Autodesk Inventor part; units mm, degrees
ref_plane "Work Plane1" through (30, 0, 0) normal (0, -0.5, 0.866) x (1, 0, 0)
ref_plane "YZ Plane" through (0, 0, 0) normal (1, 0, 0) x (0, 1, 0)
ref_plane "XZ Plane" through (0, 0, 0) normal (0, 1, 0) x (-1, 0, 0)
sketch "Sketch1" plane through (0, 0, 0) normal (0, 0, 1) x (1, 0, 0)
  line L0 (-0.6667, 0) -> (30, 0)
  line L1 (30, 0) -> (30, 1.5)
  line L2 (30, 1.5) -> (12, 1.5)
  line L3 (12, 1.5) -> (11.6933, 1.5)
  line L4 (11.6933, 1.5) -> (0, 1.5)
  line L5 (0, 1.5) -> (0, 2.75)
  line L6 (0, 2.75) -> (-3, 2.75)
  line L7 (-3, 2.75) -> (-3, 1.4434)
  line L8 (-3, 1.4434) -> (-1.5, 1.4434)
  line L9 (-1.5, 1.4434) -> (-0.6667, 0)
  line L10 (-9.6, 0) -> (36.6, 0)
  line L11 (0, -0.55) -> (0, 3.3)
  line L12 (12, 1.5) -> (0, 1.5) construction
  dimension "d0" = 18
  dimension "d1" = 0.3067
  dimension "d2" = 3
  dimension "d3" = 1.5
  dimension "d4" = 60
  dimension "d5" = 3
  dimension "d6" = 3
  dimension "d7" = 2.8868
  dimension "d8" = 5.5
  dimension "d19" = 30
revolve "Body" add sketch "Sketch1" angle 360 about axis through (-0.6667, 0, 0) along (1, 0, 0)
sketch "Sketch2" plane through (-3, 0, 0) normal (-1, 0, 0) x (0, 0, 1)
  circle A0 centre (0, 0) radius 1.4434
  line L0 (0, -3.85) -> (0, 3.85)
  line L1 (-3.85, 0) -> (3.85, 0)
  line L2 (1.4434, 0) -> (0.7217, -1.25)
  line L3 (0.7217, -1.25) -> (-0.7217, -1.25)
  line L4 (-0.7217, -1.25) -> (-1.4434, 0)
  line L5 (-1.4434, 0) -> (-0.7217, 1.25)
  line L6 (-0.7217, 1.25) -> (0.7217, 1.25)
  line L7 (0.7217, 1.25) -> (1.4434, 0)
extrude "Slot" add sketch "Sketch2" against normal up to next contours L7 A0 | A0 L2 | L6 L0 A0 | A0 L0 L3 | L0 L6 A0 | A0 L3 L0 | L4 A0 | A0 L5
fillet "Fillet2" radius 0.3 1 edges at (-3, -2.75, 0)
thread "Thread"
chamfer "Chamfer1" distance 0.3067 distance2 0.3067 1 edges at (30, -1.5, 0) measured on face at (30, -0.3888, 0.2119)
fillet "Fillet1" radius 0.1 1 edges at (0, -1.5, 0)
ref_plane "Work Plane1" through (30, 0, 0) normal (0, -0.5, 0.866) x (1, 0, 0)
equation "\"d0\" = GEL"
equation "\"d1\" = GAL"
equation "\"d2\" = KOH"
equation "\"d3\" = INTI"
equation "\"d5\" = GD"
equation "\"d6\" = BDM"
equation "\"d7\" = 1.1547 * SW"
equation "\"d8\" = KOD"
equation "\"d19\" = NLG"
equation "\"d16\" = RR"
equation "\"d12\" = GEL"
equation "\"d14\" = -0.5 * SPD + 0.5 * GD"
equation "\"d15\" = GUL"
equation "\"d29\" = R"
equation "\"GD\" = NND"
equation "\"NLG\" = 30"
equation "\"GEL\" = 18"
equation "\"KOD\" = 5.5"
equation "\"KOH\" = 3"
equation "\"INTI\" = 1.5"
equation "\"GAL\" = 0.61345 * PTC"
equation "\"GUL\" = 0.61345 * PTC"
equation "\"BDM\" = NND"
equation "\"SW\" = 2.5"
equation "\"RR\" = 0.3"
equation "\"SPD\" = 2.38655"
equation "\"d28\" = R"
equation "\"R\" = 0.1"
equation "\"TOA\" = 30deg"
equation "\"THREADDIA\" = 3"
equation "\"KOD1\" = KOD"
equation "\"PTC\" = 0.5"
equation "\"NND\" = 3"
equation "\"E0\" = 1.155 * SW"
equation "\"GD1\" = THREADDIA - 1.2269 * PTC"
properties part number "ANSI B18.3.1M - M3x0.5 x 30" material "Steel, Mild"
Geometry check sheet. Reference: the model listing, model coordinates, mm. A direction names the side the tool comes from. Round coordinates to 2 decimals unless told otherwise and drop trailing zeros.
Item 1: Go/stop test with flat-tipped pins: pin 1 Ø1 at (x, z) = (9, -1.5) entering from -Y; pin 2 Ø2 at (x, z) = (0.5, -1.5) entering from -Y; pin 3 Ø3 at (x, z) = (15.5, 0.5) entering from -Y. Record where each tip stops, or that it passes through.
Determined:
pin 1: stops at y = -1.12
pin 2: stops at y = -2.68
pin 3: stops at y = -1.5
Item 2: Mould release check, pull along Z, two halves, no side actions. Record for faces 4 (the face through (-2.205, 0.616, -1.088)), 5 (the face through (-3, -1.1, 1.1)), 6 (the face through (14.69, -1.5, -0.07)): +Z half, -Z half, draft (parallel to the pull), parting line (faces both ways), or undercut.
Determined:
face 4: undercut
face 5: draft
face 6: parting line
Item 3: Material ranges on line 1 along X through (y, z) = (-0.3, -1.9); line 2 along Y through (x, z) = (11.5, -0.1); line 3 along Z through (x, y) = (16.5, -0.15), recorded low to high.
Determined:
line 1: x = -3 to 0
line 2: y = -1.5 to 1.5
line 3: z = -1.49 to 1.49
Item 4: Access from +Z, -Z, +X, -X, +Y, -Y to the whole of each face (thin tool, end or side, straight path). Record for faces 1 (the face through (30, 0, 0)), 2 (the face through (0, 2, 0)), 3 (the face through (-2.21, -0.63, -1.08)).
Determined:
face 1: +Z, -Z, +X, +Y, -Y
face 2: +X
face 3: -X
